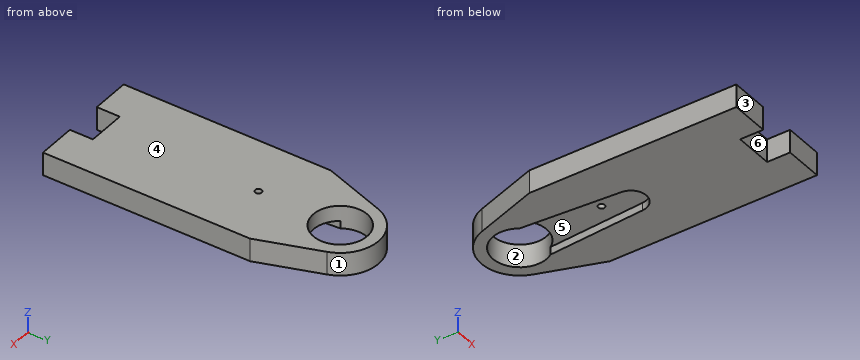
from build123d import *

# Parameters (mm, degrees)
CORTE_EXTERIOR_R        = 0.425
CORTE_EXTERIOR_R_2      = 3.500002336
SALIENTE_EXTRUIR1_DEPTH = 3
CORTAR_EXTRUIR1_DEPTH   = 1


with BuildPart() as part:
    # Corte exterior → Saliente-Extruir1 (new body)
    with BuildSketch(Plane.XY):
        with BuildLine():
            Line((40.01577693, -3.310783785), (40.01577693, 10.689216215))
            Line((40.01577693, 10.689216215), (40.01577693, 23.689216215))
            Line((40.01577693, 23.689216215), (37.248055694, 31.80338402))
            ThreePointArc((37.248055694, 31.80338402), (32.51577693, 35.189216215), (27.783498166, 31.80338402))
            Line((27.783498166, 31.80338402), (25.01577693, 23.689216215))
            Line((25.01577693, 23.689216215), (25.01577693, -3.310783785))
            Line((25.01577693, -3.310783785), (30.01577693, -3.310783785))
            Line((30.01577693, -3.310783785), (30.01577693, -0.310783785))
            Line((30.01577693, -0.310783785), (35.01577693, -0.310783785))
            Line((35.01577693, -0.310783785), (35.01577693, -3.310783785))
            Line((35.01577693, -3.310783785), (40.01577693, -3.310783785))
        make_face()
        with Locations((32.51577693, 19.516986762)):
            Circle(CORTE_EXTERIOR_R, mode=Mode.SUBTRACT)
        with Locations((32.51577693, 30.189216215)):
            Circle(CORTE_EXTERIOR_R_2, mode=Mode.SUBTRACT)
    extrude(amount=SALIENTE_EXTRUIR1_DEPTH)

    # Grabado Superficie → Cortar-Extruir1 (cut)
    with BuildSketch(Plane.XY):
        with BuildLine():
            Line((30.520602357, 15.55036945), (29.64077693, 28.193122191))
            ThreePointArc((29.64077693, 28.193122191), (32.51577693, 26.689213879), (35.39077693, 28.193122191))
            Line((35.39077693, 28.193122191), (34.510951503, 15.55036945))
            ThreePointArc((34.510951503, 15.55036945), (32.51577693, 13.689216215), (30.520602357, 15.55036945))
        make_face()
    extrude(amount=CORTAR_EXTRUIR1_DEPTH, mode=Mode.SUBTRACT)


solid = part.part
Design review of the part built by this model. Coordinates are the model's own, in mm. Face numbers are marked on the shaded views. A direction names the side the tool comes from. Give positions to 0.01 mm unless a question says otherwise; leave off trailing zeros. Order: outer loops, then holes, each group sorted by start corner. A loop starts at its lowest first (then second) coordinate and runs counter-clockwise, first axis right, second up. Notation, with made-up numbers: (1.25, 35) - (14.25, 35) arc R26 ccw to (14.25, 51) - close; hole circle Ø1 at (50, 64). An arc over 180 degrees is marked (long way). Write item = value, one per line. Start each with the question number.
Q1. Tool access review of the marked faces 4, 5 and 6: name each direction out of +Z, -Z, +X, -X, +Y, -Y from which nothing blocks a thin tool from reaching the whole face with its end or side.
Q2. We need section A-A on x = 31. State the section outline as (y, z) points.
Q3. Mouldability with a two-part tool opening along X and no side actions: class the marked faces 1, 2 and 3 as released by +X, released by -X, zero draft, split by the parting line, or undercut.
Q4. To check wall thickness, follow L1, parallel to Y at x = 34, z = 0.85; L2, parallel to X at y = 30, z = 0.25; L3, parallel to X at y = 16, z = 0.8. State the ranges of each line that lie inside material, in increasing order. Write a range as from..to.
Q5. We need section B-B on z = 0.65. State the section outline as (x, y) points, plus the area to 3 significant figures.
Q6. We need section C-C on x = 32.5. State the section outline as (y, z) points, plus the area to 3 significant figures.
Q7. We need section D-D on y = 17.5. State the section outline as (x, z) points, plus the area to 3 significant figures.
Working result:
q1.face_4 = +Z, +X, -X, +Y, -Y
q1.face_5 = -Z
q1.face_6 = +Z, -Z, -Y
q2.outline = (-0.31, 0) - (14.38, 0) - (14.38, 1) - (27.03, 1) - (27.03, 3) - (-0.31, 3) - close; (33.34, 0) - (34.95, 0) - (34.95, 3) - (33.34, 3) - close
q3.face_1 = split by the parting line
q3.face_2 = undercut
q3.face_3 = zero draft
q4.L1 = -0.31..14.35, 33.36..34.96
q4.L2 = 27.17..29.02, 36.01..37.86
q4.L3 = 25.02..30.49, 34.54..40.02
q5.outline = (25.02, -3.31) - (30.02, -3.31) - (30.02, -0.31) - (35.02, -0.31) - (35.02, -3.31) - (40.02, -3.31) - (40.02, 23.69) - (37.25, 31.8) arc R5 ccw to (27.78, 31.8) - (25.02, 23.69) - close; hole (29.64, 28.19) - (30.52, 15.55) arc R2 ccw to (34.51, 15.55) - (35.39, 28.19) arc R3.5 ccw (long way) to start
q5.area = 413 mm²
q6.outline = (-0.31, 0) - (13.69, 0) - (13.69, 1) - (19.09, 1) - (19.09, 3) - (-0.31, 3) - close; (19.94, 1) - (26.69, 1) - (26.69, 3) - (19.94, 3) - close; (33.69, 0) - (35.19, 0) - (35.19, 3) - (33.69, 3) - close
q6.area = 70.8 mm²
q7.outline = (25.02, 0) - (30.38, 0) - (30.38, 1) - (34.65, 1) - (34.65, 0) - (40.02, 0) - (40.02, 3) - (25.02, 3) - close
q7.area = 40.7 mm²
